Can you work these out from the model? Positions are in its coordinate system, mm. A direction names the side the tool comes from. Coordinates: 2 decimals unless noted, no trailing zeros. Loops run counter-clockwise (first coordinate to the right, second up) from the corner with the lowest first, then second, coordinate; pieces in that order, holes last. Notation, with made-up numbers: (59.25, 14.5) -> (65.25, 14.5) arc R37 ccw to (65.25, 52.5) -> close; hole circle Ø5 at (87, 53). An arc over 180 degrees is marked (long way). Put each result on its own line as item: value. Start each with the question number.
Item 1: If we section it at D-D on x = 25: Please give me the cut outline in (y, z).
Item 2: If we section it at A-A on y = 0: Please give me the cut outline in (x, z).
Item 3: For faces 5 (the flat face through (39, 4, -4)), 6 (the flat face through (12, 1, -3)), 7 (the flat face through (39, -4, -4)), 8 (the flat face through (55, 0, -4.5)), which set-ups out of +Z, -Z, +X, -X, +Y, -Y let a thin tool reach every point of the face, with its end or its side?
Item 4: Please list where these lines run through material, in increasing order: L1, parallel to Y at x = 0, z = -0.75; L2, parallel to Y at x = 60, z = -5.4; L3, parallel to X at y = 5, z = -2.25. Write a range as from..to.
Item 5: We'd pull the mould along Y, two halves only. Please class faces 1 (the cylindrical face through (13.32, -4.97, -1.48)), 2 (the cylindrical face through (64, 0, -6)), 3 (the flat face through (37.89, -0.06, -5.22)), 4 (the cylindrical face through (-2.38, -10.74, -1.48)): pulls with the +Y half, pulls with the -Y half, needs draft (parallel to the pull), parting line crosses it, or undercut.
Item 6: Will these pins go through, and if not, where does the flat tip stop? P1, Ø8, axis at x = 60, y = 0, coming from the +Z side; P2, Ø4, axis at y = 8, z = -1.5, coming from the -X side; P3, Ø4, axis at y = 10, z = -3, coming from the -X side.
Item 7: If we section it at C-C on z = -1.5: Please give me the cut outline in (x, y).
Item 8: If we section it at B-B on y = 6.5: Please give me the cut outline in (x, z).
Autodesk Inventor part; units mm, degrees
ref_plane "Work Plane3" through (0, 0, 0) normal (0, 1, 0) x (-1, 0, 0)
ref_plane "YZ Plane" through (0, 0, 0) normal (1, 0, 0) x (0, 1, 0)
ref_plane "XY Plane" through (0, 0, 0) normal (0, 0, 1) x (1, 0, 0)
sketch "Sketch1" plane through (0, 0, 0) normal (0, 0, 1) x (1, 0, 0)
  arc A0 (9.7855, 7.7778) -> (9.7855, -7.7778) centre (0, 0) ccw
  circle A1 centre (0, 0) radius 11
  arc A2 (60, -4) -> (60, 4) centre (60, 0) ccw
  line L0 (60, 4) -> (17.6139, 4) construction
  line L1 (60, -4) -> (17.6139, -4) construction
  arc A3 (17.6139, -4) -> (9.7855, -7.7778) centre (17.6139, -14) ccw
  arc A4 (9.7855, 7.7778) -> (17.6139, 4) centre (17.6139, 14) ccw
  line L2 (30, 4) -> (30, -4) construction
  line L3 (17.6139, -4) -> (17.6139, 4)
  point P0 (11.8427, 4)
  point P1 (11.8427, -4)
  point P2 (-12.5, 0)
  point P3 (30, 0)
  dimension "d0" = 25
  dimension "d1" = 22
  dimension "d2" = 4
  dimension "d3" = 10
  dimension "d4" = 60
  dimension "d17" = 42.5
extrude "Extrusion1" add sketch "Sketch1" against normal blind 3
ref_plane "Work Plane3" through (0, 0, 0) normal (0, 1, 0) x (-1, 0, 0)
sketch "Sketch7" plane through (0, 0, 0) normal (0, 1, 0) x (-1, 0, 0)
  line L0 (-17.6139, 0) -> (-17.6139, -3)
  line L1 (-17.6139, -3) -> (-30, -3)
  line L2 (-30, -3) -> (-46, -7.5)
  line L3 (-46, -7.5) -> (-60, -7.5)
  line L4 (-60, -7.5) -> (-60, -4.5)
  line L5 (-60, -4.5) -> (-46, -4.5)
  line L6 (-46, -4.5) -> (-30, 0)
  line L7 (-30, 0) -> (-17.6139, 0)
  line L8 (-17.6139, -3) -> (-17.6139, 0)
  point P0 (0, 0)
  point P1 (-60, -6)
  dimension "d19" = 4.5
  dimension "d20" = 14
  dimension "d21" = 60
  dimension "d22" = 3
extrude "Extrusion3" add sketch "Sketch7" along normal mid plane 8
sketch "Sketch8" plane through (46, 4, -4.5) normal (0, 0, 1) x (1, 0, 0)
  line L0 (14, -8) -> (14, 0)
  arc A0 (14, -8) -> (14, 0) centre (14, -4) ccw
  point P0 (-46, -4)
  dimension "d25" = 4
extrude "Extrusion4" add sketch "Sketch8" against normal up to surface (3 mm away)
sketch "Sketch9" plane through (46, -4, -4.5) normal (0, 0, 1) x (1, 0, 0)
  arc A0 (14, 0) -> (14, 8) centre (14, 4) ccw
  point P0 (-46, 4)
hole "Hole1" at (60, 0, -4.5) direction (0, 0, -1) diameter 5 depth 3
properties part number "15_2"
Solutions:
1. outline: (-4, -3) -> (4, -3) -> (4, 0) -> (-4, 0) -> close
2. outline: (-12.5, -3) -> (-11, -3) -> (-11, 0) -> (-12.5, 0) -> close; (11, -3) -> (30, -3) -> (46, -7.5) -> (57.5, -7.5) -> (57.5, -4.5) -> (46, -4.5) -> (30, 0) -> (11, 0) -> close; (62.5, -7.5) -> (64, -7.5) -> (64, -4.5) -> (62.5, -4.5) -> close
3. face 5: +Z, -Z, +X, +Y
3. face 6: -Z, -X, +Y, -Y
3. face 7: +Z, -Z, +X, -Y
3. face 8: +Z, +X, +Y, -Y
4. L1: -12.5..-11, 11..12.5
4. L2: -4..-2.5, 2.5..4
4. L3: -11.46..-9.8, 9.8..13.26
5. face 1: pulls with the -Y half
5. face 2: parting line crosses it
5. face 3: needs draft
5. face 4: undercut
6. P1: z = -4.5
6. P2: x = -10.97
6. P3: x = -9.6
7. outline: (9.79, -7.78) arc R10 cw to (17.61, -4) -> (35.33, -4) -> (35.33, 4) -> (17.61, 4) arc R10 cw to (9.79, 7.78) arc R12.5 ccw (long way) to start; hole circle Ø22 at (0, 0)
8. outline: (-10.68, -3) -> (-8.87, -3) -> (-8.87, 0) -> (-10.68, 0) -> close; (8.87, -3) -> (11, -3) -> (11, 0) -> (8.87, 0) -> close
